Can you work these out from the model? Positions are in its coordinate system, mm. Face numbers are marked on the shaded views. A direction names the side the tool comes from. Give positions to 0.01 mm unless a question says otherwise; leave off trailing zeros. Loops run counter-clockwise (first coordinate to the right, second up) from the corner with the lowest first, then second, coordinate; pieces in that order, holes last. Notation, with made-up numbers: (22, -11.75) - (40, -11.75) arc R25 ccw to (40, 5.25) - close; hole circle Ø3 at (61, 46.5). An arc over 180 degrees is marked (long way). Use a Markdown table: item, result. Add a question column.
```python
from build123d import *

# Parameters (mm, degrees)
F1_DEPTH = 7.62
F2_R     = 1.5875
F3_R     = 1.5875
F4_DEPTH = 25.4
F2_R_2   = 2.921
F3_R_2   = 2.921
F5_DEPTH = 2.794
F6_ANGLE = -90


with BuildPart() as f1:
    # F0 (on Top) → F1 (new body)
    with BuildSketch(Plane.XY):
        with BuildLine():
            Line((11.43, 1.27), (12.6363404513, 1.27))
            ThreePointArc((12.6363404513, 1.27), (12.2207385876, 3.4559439194), (11.43, 5.5358016583))
            Line((11.43, 5.5358016583), (11.43, 1.27))
        make_face()
        with BuildLine():
            ThreePointArc((11.43, 5.5358016583), (12.2207385876, 3.4559439194), (12.6363404513, 1.27))
            Line((12.6363404513, 1.27), (19.05, 1.27))
            Line((19.05, 1.27), (19.05, 7.62))
            Line((19.05, 7.62), (11.43, 7.62))
            Line((11.43, 7.62), (11.43, 5.5358016583))
        make_face()
        with BuildLine():
            Line((11.43, 1.27), (11.43, 5.5358016583))
            ThreePointArc((11.43, 5.5358016583), (10.8451830635, 6.6084797282), (10.16, 7.62))
            Line((10.16, 7.62), (-10.16, 7.62))
            ThreePointArc((-10.16, 7.62), (-10.8451830635, 6.6084797282), (-11.43, 5.5358016583))
            Line((-11.43, 5.5358016583), (-11.43, 1.27))
            Line((-11.43, 1.27), (-6.8685751798, 1.27))
            ThreePointArc((-6.8685751798, 1.27), (0, 6.985), (6.8685751798, 1.27))
            Line((6.8685751798, 1.27), (11.43, 1.27))
        make_face()
        with BuildLine():
            ThreePointArc((10.16, 7.62), (10.8451830635, 6.6084797282), (11.43, 5.5358016583))
            Line((11.43, 5.5358016583), (11.43, 7.62))
            Line((11.43, 7.62), (10.16, 7.62))
        make_face()
        with BuildLine():
            Line((-10.16, 7.62), (10.16, 7.62))
            ThreePointArc((10.16, 7.62), (0, 12.7), (-10.16, 7.62))
        make_face()
        with BuildLine():
            ThreePointArc((-11.43, 5.5358016583), (-10.8451830635, 6.6084797282), (-10.16, 7.62))
            Line((-10.16, 7.62), (-11.43, 7.62))
            Line((-11.43, 7.62), (-11.43, 5.5358016583))
        make_face()
        with BuildLine():
            Line((-11.43, 1.27), (-11.43, 5.5358016583))
            ThreePointArc((-11.43, 5.5358016583), (-12.2207385876, 3.4559439194), (-12.6363404513, 1.27))
            Line((-12.6363404513, 1.27), (-11.43, 1.27))
        make_face()
        with BuildLine():
            ThreePointArc((-12.6363404513, 1.27), (-12.2207385876, 3.4559439194), (-11.43, 5.5358016583))
            Line((-11.43, 5.5358016583), (-11.43, 7.62))
            Line((-11.43, 7.62), (-19.05, 7.62))
            Line((-19.05, 7.62), (-19.05, 1.27))
            Line((-19.05, 1.27), (-12.6363404513, 1.27))
        make_face()
    extrude(amount=F1_DEPTH)

    # F2 (on face) + F3 (on face) → F4 (cut)
    with BuildSketch(Plane(origin=(0, 7.62, 0), x_dir=(-1, 0, 0), z_dir=(0, 1, 0))):
        with Locations((-15.24, 3.81)):
            Circle(F2_R)
    with BuildSketch(Plane(origin=(0, 7.62, 0), x_dir=(-1, 0, 0), z_dir=(0, 1, 0))):
        with Locations((15.24, 3.81)):
            Circle(F3_R)
    extrude(amount=-F4_DEPTH, mode=Mode.SUBTRACT)

    # F2 (on face) + F3 (on face) → F5 (cut)
    with BuildSketch(Plane(origin=(0, 7.62, 0), x_dir=(-1, 0, 0), z_dir=(0, 1, 0))):
        with Locations((-15.24, 3.81)):
            Circle(F2_R_2)
        with Locations((-15.24, 3.81)):
            Circle(F2_R, mode=Mode.SUBTRACT)
    with BuildSketch(Plane(origin=(0, 7.62, 0), x_dir=(-1, 0, 0), z_dir=(0, 1, 0))):
        with Locations((15.24, 3.81)):
            Circle(F3_R_2)
        with Locations((15.24, 3.81)):
            Circle(F3_R, mode=Mode.SUBTRACT)
    extrude(amount=-F5_DEPTH, mode=Mode.SUBTRACT)


with BuildPart() as f1_1:
    # F6: moved
    add(f1.part.rotate(Axis((19.05, 7.62, 3.81), (0, 0, -1)), F6_ANGLE))


solid = f1_1.part
```
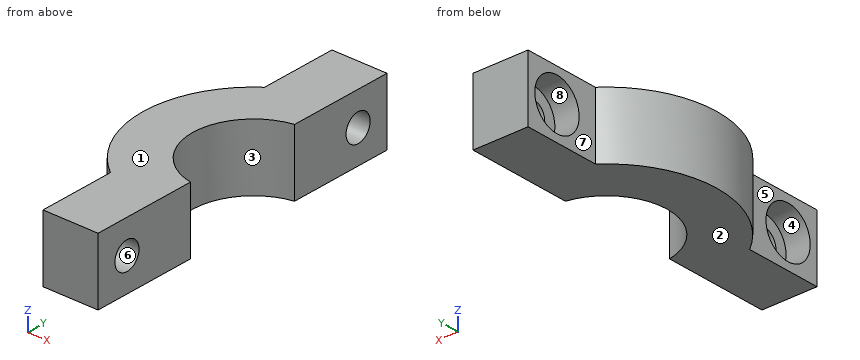
1. Please list where these lines run through material, in increasing order: line 1 along Z through (x, y) = (20.9, -26.67); line 2 along Z through (x, y) = (23.9, 3.81); line 3 along Y through (x, z) = (21.5, 1.5). Write a range as [from, to].
2. Suppose I cut it at B-B (y = -26.67). List the corners of the cut face in (x, z) for me.
3. Suppose I cut it at A-A (z = 3.81). State how many separate pieces and enclosed holes the cut face has, and give its area (3 significant figures).
4. Will these pins go through, and if not, where does the flat tip stop? P1, Ø1.8, axis at y = -25.5, z = 2.5, coming from the -X side; P2, Ø2.5, axis at y = 3.81, z = 3.81, coming from the -X side; P3, Ø3, axis at y = -14.5, z = 3, coming from the +X side; P4, Ø5, axis at x = 20.5, y = -14, coming from the -Z side.
5. Suppose I cut it at C-C (z = 1.5). List the corners of the cut face in (x, y) for me (3 decimals).
6. On a 3-axis mill with a long thin cutter (end or side, diameter ignored), from which of +Z, -Z, +X, -X, +Y, -Y can I reach the whole of each face in a straight line? I mean the marked faces 5, 6, 7 and 8. Say none if no direction works.
7. Suppose I cut it at D-D (x = 15.5). List the corners of the cut face in (y, z) for me, and give its area (3 significant figures).
8. If we mould it in two halves opening along Z, with no side actions, what happens to the marked faces 1, 2, 3 and 4? For each: released by +Z, released by -Z, zero draft, split by the parting line, or undercut.
Results below:
| question | item | result |
|---|---|---|
| 1 | line 1 | [0, 0.89], [6.73, 7.62] |
| 1 | line 2 | [0, 2.22], [5.4, 7.62] |
| 1 | line 3 | [-30.48, -28.46], [-24.88, -16.13], [-6.73, 2.02], [5.6, 7.62] |
| 2 | outline | (19.05, 0) - (25.4, 0) - (25.4, 2.22) - (21.84, 2.22) - (21.84, 0.89) - (19.05, 0.89) - close; (19.05, 6.73) - (21.84, 6.73) - (21.84, 5.4) - (25.4, 5.4) - (25.4, 7.62) - (19.05, 7.62) - close |
| 3 | separate pieces | 3 |
| 3 | enclosed holes | 0 |
| 3 | area | 200 mm² |
| 4 | P1 | x = 21.84 |
| 4 | P2 | through |
| 4 | P3 | x = 21.39 |
| 4 | P4 | z = 0 |
| 5 | outline | (19.05, -30.48) - (25.4, -30.48) - (25.4, -18.299) arc R6.985 cw to (25.4, -4.561) - (25.4, 7.62) - (19.05, 7.62) - (19.05, 5.598) - (21.844, 5.598) - (21.844, 2.022) - (19.05, 2.022) - (19.05, -1.27) arc R12.7 ccw to (19.05, -21.59) - (19.05, -24.882) - (21.844, -24.882) - (21.844, -28.458) - (19.05, -28.458) - close |
| 6 | face 5 | +Z, -Z, -X, -Y |
| 6 | face 6 | +X, -X |
| 6 | face 7 | +Z, -Z, -X, +Y |
| 6 | face 8 | -X |
| 7 | outline | (-17.47, 0) - (-5.39, 0) - (-5.39, 7.62) - (-17.47, 7.62) - close |
| 7 | area | 92.1 mm² |
| 8 | face 1 | released by +Z |
| 8 | face 2 | released by -Z |
| 8 | face 3 | zero draft |
| 8 | face 4 | undercut |
